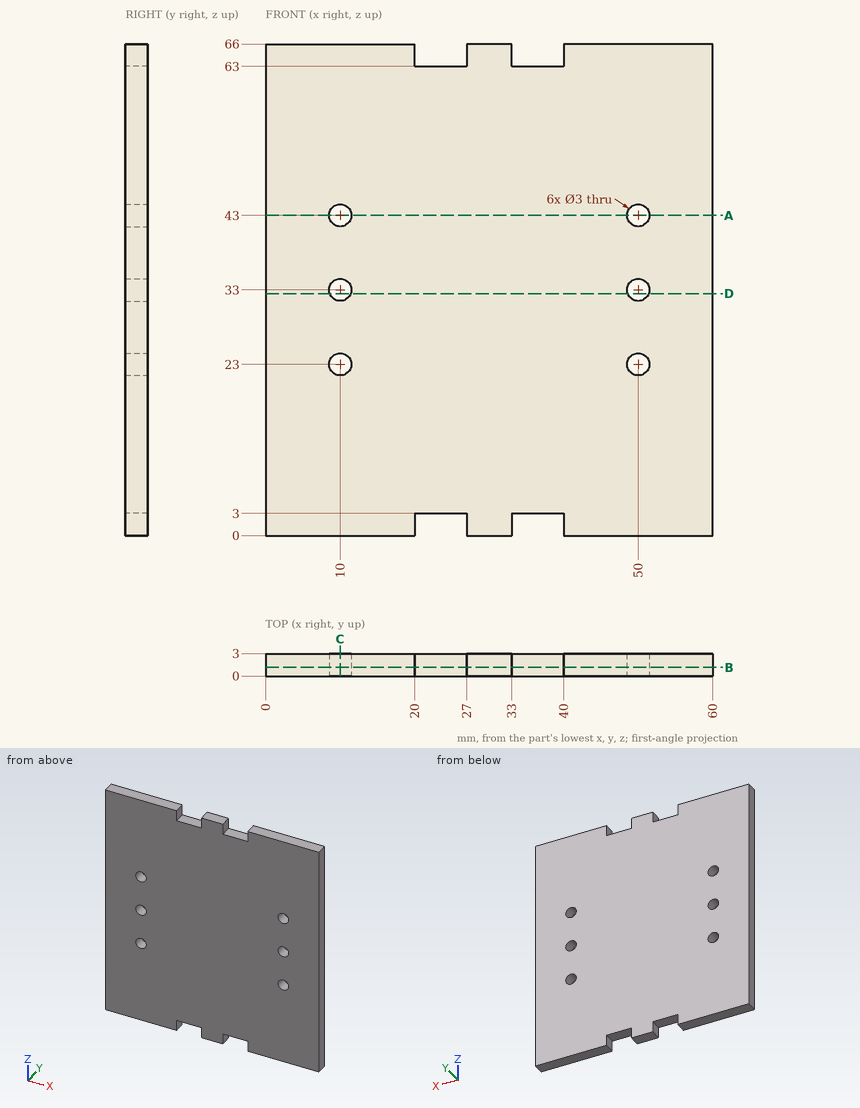
Answer from the drawing. Dimensions are ordinates in mm from the lowest x, y and z of the part. Give positions to 0.01 mm unless a question says otherwise; leave off trailing zeros. Order: outer loops, then holes, each group sorted by start corner. A loop starts at its lowest first (then second) coordinate and runs counter-clockwise, first axis right, second up. Notation, with made-up numbers: (-7, 60) -> (32, 60) arc R28 cw to (32, 98) -> close; hole circle Ø1 at (71, 18). An arc over 180 degrees is marked (long way). One line per item, written item: value.
Item 1: Find section D-D, the plane z = 32.5. Give the vertices of the cut face in (x, y).
Answer sheet:
outline: (0, 0) -> (8.59, 0) -> (8.59, 3) -> (0, 3) -> close; (11.41, 0) -> (48.59, 0) -> (48.59, 3) -> (11.41, 3) -> close; (51.41, 0) -> (60, 0) -> (60, 3) -> (51.41, 3) -> close
Item 2: Find section C-C, the plane x = 10. Give the vertices of the cut face in (y, z), plus the area to 3 significant figures.
Answer sheet:
outline: (0, 0) -> (3, 0) -> (3, 21.5) -> (0, 21.5) -> close; (0, 24.5) -> (3, 24.5) -> (3, 31.5) -> (0, 31.5) -> close; (0, 34.5) -> (3, 34.5) -> (3, 41.5) -> (0, 41.5) -> close; (0, 44.5) -> (3, 44.5) -> (3, 66) -> (0, 66) -> close
area: 171 mm²
Item 3: Find section B-B, the plane y = 1.15. Give the vertices of the cut face in (x, z), plus the area to 3 significant figures.
Answer sheet:
outline: (0, 0) -> (20, 0) -> (20, 3) -> (27, 3) -> (27, 0) -> (33, 0) -> (33, 3) -> (40, 3) -> (40, 0) -> (60, 0) -> (60, 66) -> (40, 66) -> (40, 63) -> (33, 63) -> (33, 66) -> (27, 66) -> (27, 63) -> (20, 63) -> (20, 66) -> (0, 66) -> close; hole circle Ø3 at (10, 23); hole circle Ø3 at (10, 33); hole circle Ø3 at (10, 43); hole circle Ø3 at (50, 23); hole circle Ø3 at (50, 33); hole circle Ø3 at (50, 43)
area: 3,830 mm²
Item 4: Straight lines are drawn through the part: probe 1 along X at (y, z) = (1, 23); probe 2 along Z at (x, y) = (50, 2.3); probe 3 along Z at (x, y) = (26.5, 1.35). For each, find the intervals that lie inside material, in ascending order.
Answer sheet:
probe 1: 0 to 8.5, 11.5 to 48.5, 51.5 to 60
probe 2: 0 to 21.5, 24.5 to 31.5, 34.5 to 41.5, 44.5 to 66
probe 3: 3 to 63
Item 5: Find section A-A, the plane z = 43. Give the vertices of the cut face in (x, y), plus the area to 3 significant figures.
Answer sheet:
outline: (0, 0) -> (8.5, 0) -> (8.5, 3) -> (0, 3) -> close; (11.5, 0) -> (48.5, 0) -> (48.5, 3) -> (11.5, 3) -> close; (51.5, 0) -> (60, 0) -> (60, 3) -> (51.5, 3) -> close
area: 162 mm²
Item 6: Flat-ended cylindrical pins translate along their axes: P1, Ø1.5, axis at x = 23.5, y = 1, coming from the +Z side; P2, Ø1.8, axis at x = 50, z = 33, coming from the -Y side. Find the tip coordinate at first contact, or state that the pin passes through.
Answer sheet:
P1: z = 63
P2: through
